from build123d import *

# Parameters (mm, degrees)
SZKIC1_R                    = 7
DODANIE_WYCI_GNI_CIE1_DEPTH = 5
SZKIC2_W                    = 50
SZKIC2_H                    = 25
DODANIE_WYCI_GNI_CIE2_DEPTH = 1000
SZKIC3_R                    = 7
DODANIE_WYCI_GNI_CIE3_DEPTH = 5
ZAOKR_GLENIE1_R             = 5
ZAOKR_GLENIE2_R             = 5
ZAOKR_GLENIE3_R             = 5
ZAOKR_GLENIE4_R             = 5


with BuildPart() as part:
    # Szkic1 → Dodanie-wyciągnięcie1 (new body)
    with BuildSketch(Plane.XY):
        Polygon((0, 0), (100, 0), (114.43375673, -25), (-14.43375673, -25), align=None)
        with Locations((93.301270189, -11.602540378)):
            Circle(SZKIC1_R, mode=Mode.SUBTRACT)
        with Locations((6.698729811, -11.602540378)):
            Circle(SZKIC1_R, mode=Mode.SUBTRACT)
    extrude(amount=DODANIE_WYCI_GNI_CIE1_DEPTH)

    # Szkic2 → Dodanie-wyciągnięcie2 (add)
    with BuildSketch(Plane.XY.offset(5)):
        with Locations((50, -12.5)):
            Rectangle(SZKIC2_W, SZKIC2_H)
    extrude(amount=DODANIE_WYCI_GNI_CIE2_DEPTH)

    # Szkic3 → Dodanie-wyciągnięcie3 (add)
    with BuildSketch(Plane.XY.offset(1005)):
        Polygon((-14.43375673, -25), (25, -25), (75, -25), (114.43375673, -25), (100, 0), (75, 0), (25, 0), (0, 0), align=None)
        with Locations((93.301270189, -11.602540378)):
            Circle(SZKIC3_R, mode=Mode.SUBTRACT)
        with Locations((6.698729811, -11.602540378)):
            Circle(SZKIC3_R, mode=Mode.SUBTRACT)
    extrude(amount=DODANIE_WYCI_GNI_CIE3_DEPTH)

    # Zaokrąglenie1
    zaokr_glenie1_edges = [part.edges().sort_by_distance(p)[0] for p in [
        (25, -12.5, 5),
    ]]
    fillet(zaokr_glenie1_edges, radius=ZAOKR_GLENIE1_R)

    # Zaokrąglenie2
    zaokr_glenie2_edges = [part.edges().sort_by_distance(p)[0] for p in [
        (75, -12.5, 5),
    ]]
    fillet(zaokr_glenie2_edges, radius=ZAOKR_GLENIE2_R)

    # Zaokrąglenie3
    zaokr_glenie3_edges = [part.edges().sort_by_distance(p)[0] for p in [
        (75, -12.5, 1005),
    ]]
    fillet(zaokr_glenie3_edges, radius=ZAOKR_GLENIE3_R)

    # Zaokrąglenie4
    zaokr_glenie4_edges = [part.edges().sort_by_distance(p)[0] for p in [
        (25, -12.5, 1005),
    ]]
    fillet(zaokr_glenie4_edges, radius=ZAOKR_GLENIE4_R)


solid = part.part
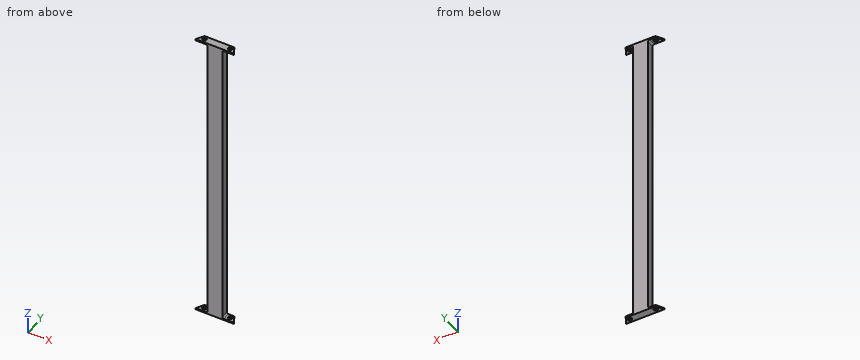
Work out the finished part from the listing and answer in its coordinate system (mm). Give positions to 0.01 mm unless a question says otherwise; leave off trailing zeros. Write each loop counter-clockwise with the first axis right and the second up, starting at its lowest first coordinate (ties: lowest second). Pieces come first, ordered by that corner, then holes. Notation, with made-up numbers: (60, 7) - (95, 7) arc R13 cw to (95, 32) - close; hole circle Ø8 at (79.25, -33). An arc over 180 degrees is marked (long way). One line per item, written item: value. Start each with the question number.
1. Find section A-A (z = 546). Write down the section's boundary in (x, y), then the cut area to 3 significant figures.
2. Given pin 1 (12 mm diameter, centred on y = -21, z = 708.5, fed in from -X); pin 2 (2 mm diameter, centred on y = -4, z = 769.5, fed in from +X), each flat-ended and moving along its own axis, determine where each tip first touches the part or whether it passes through.
3. Consider probe 1 along Z at (x, y) = (84.5, -13.5); probe 2 along X at (y, z) = (-21.75, 725). Determine where each line is inside the solid, lowest interval first.
Geometry results:
1. outline: (25, -25) - (75, -25) - (75, 0) - (25, 0) - close
1. area: 1,250 mm2
2. pin 1: x = 25
2. pin 2: x = 75
3. probe 1: 0 to 5, 1005 to 1010
3. probe 2: 25 to 75
